Input: part model. Units: mm. Frame: model coordinates. Face numbers are marked on the shaded views. A direction names the side the tool comes from. Coordinates: 2 decimals unless noted, no trailing zeros. Loops run counter-clockwise (first coordinate to the right, second up) from the corner with the lowest first, then second, coordinate; pieces in that order, holes last.
Item 1: Section A-A on z = 11.5. Return loops of the section in (x, y), and give its area (3 significant figures).
Item 2: Section B-B on y = -2.5. Return loops of the section in (x, z).
Item 3: Section D-D on z = 18.25. Return loops of the section in (x, y), and give its area (3 significant figures).
Item 4: Contact query for flat-ended pins moving along their axis: P1, Ø5, axis at y = 20, z = 14, coming from the +X side; P2, Ø1.5, axis at x = 29.5, z = 2.5, coming from the -Y side. Output: stop coordinate, or through.
Item 5: Ray query, line 1 along Y through (x, z) = (12, 13.5); line 2 along X through (y, z) = (24, 4.25); line 3 along Y through (x, z) = (-1.5, 15). Return the intervals inside material, ascending.
Item 6: Pull-direction query (Z, two-part tool) for the marked faces 1, 2 and 3; classes: released by +Z, released by -Z, zero draft, split by the parting line, or undercut.
Item 7: Reachability of the marked faces 4 and 5 from +Z, -Z, +X, -X, +Y, -Y: full face, straight path, thin tool, end or side. Return the list, or none.
Item 8: Section C-C on x = 33. Return loops of the section in (y, z).
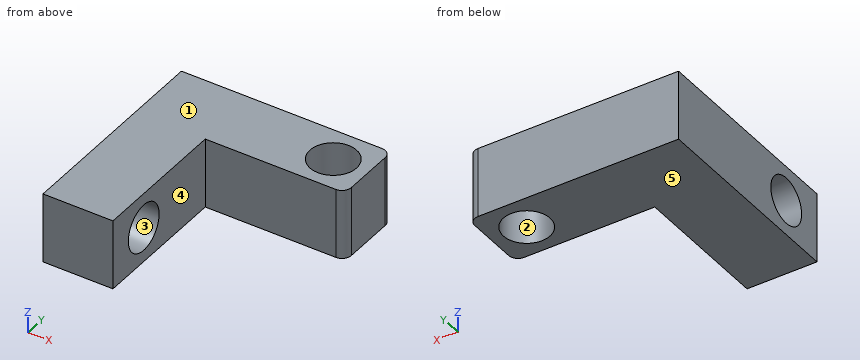
```python
from build123d import *

# Parameters (mm, degrees)
F1_DEPTH = 19.05
F3_D     = 12.7
F4_R     = 2.54
F6_D     = 12.7


# Not quite as in the source:
# - a feature names something its author has since deleted; it is built from what else it names


with BuildPart() as f1:
    # F0 (on Top) → F1 (new body)
    with BuildSketch(Plane.XY):
        Polygon((-12.7313164792, 44.4748119943), (-12.7313164792, -12.6751880057), (6.3186835208, -12.6751880057), (6.3186835208, 25.4248119943), (44.4186835208, 25.4248119943), (44.4186835208, 44.4748119943), align=None)
    extrude(amount=F1_DEPTH)

    # F3 (through all)
    with Locations(Plane.XY.offset(19.05)):
        with Locations((34.8936835208, 34.9498119943)):
            Hole(F3_D / 2)

    # F4
    f4_edges = [f1.edges().sort_by_distance(p)[0] for p in [
        (44.418684, 25.424812, 9.525),
        (44.418684, 44.474812, 9.525),
    ]]
    fillet(f4_edges, radius=F4_R)

    # F6 (through all)
    with Locations(Plane.YZ.offset(6.3186835208)):
        with Locations((0.0248119943, 9.525)):
            Hole(F6_D / 2)


solid = f1.part
```
Results found:
1. outline: (-12.73, -12.68) - (6.32, -12.68) - (6.32, -6.01) - (-12.73, -6.01) - close; (-12.73, 6.06) - (6.32, 6.06) - (6.32, 25.42) - (41.88, 25.42) arc R2.54 ccw to (44.42, 27.96) - (44.42, 41.93) arc R2.54 ccw to (41.88, 44.47) - (-12.73, 44.47) - close; hole circle Ø12.7 at (34.89, 34.95)
1. area: 1,460 mm2
2. outline: (-12.73, 0) - (6.32, 0) - (6.32, 3.7) - (-12.73, 3.7) - close; (-12.73, 15.35) - (6.32, 15.35) - (6.32, 19.05) - (-12.73, 19.05) - close
3. outline: (-12.73, -12.68) - (6.32, -12.68) - (6.32, 25.42) - (41.88, 25.42) arc R2.54 ccw to (44.42, 27.96) - (44.42, 41.93) arc R2.54 ccw to (41.88, 44.47) - (-12.73, 44.47) - close; hole circle Ø12.7 at (34.89, 34.95)
3. area: 1,690 mm2
4. P1: stops at x = 6.32
4. P2: stops at y = 25.42
5. line 1: y = 25.42 to 44.47
5. line 2: x = -12.73 to 6.32
5. line 3: y = -12.68 to -3.19, 3.24 to 44.47
6. face 1: released by +Z
6. face 2: zero draft
6. face 3: undercut
7. face 4: +Z, -Z, +X, -Y
7. face 5: -Z, +X, -X, +Y, -Y
8. outline: (25.42, 0) - (28.89, 0) - (28.89, 19.05) - (25.42, 19.05) - close; (41.01, 0) - (44.47, 0) - (44.47, 19.05) - (41.01, 19.05) - close
